Build history of the part. All positions in model axes, mm. A direction names the side the tool comes from. Round coordinates to 2 decimals unless told otherwise and drop trailing zeros. Order: outer loops, then holes, each group sorted by start corner. A loop starts at its lowest first (then second) coordinate and runs counter-clockwise, first axis right, second up. Notation, with made-up numbers: (21.5, -21) -> (48.5, -21) arc R12 ccw to (48.5, -15) -> close; hole circle Ø3 at (-4.5, 11). An arc over 180 degrees is marked (long way). Use a Markdown table: item, result. Add a question column.
Item 1: Probe L1, parallel to X at y = 3.5, z = 5; L2, parallel to Z at x = 21, y = 5.25 (3 decimals); L3, parallel to Y at x = -2.5, z = 3.5. List the from-to ranges inside material, lowest first.
Item 2: 3-axis set-ups, long thin cutter, end or side, ignore diameter. For faces 5 (the face through (2, 7.525, 2)), 6 (the face through (-2, 0, 7.264)), 7 (the face through (-27.43, 2.47, 4.58)): which of +Z, -Z, +X, -X, +Y, -Y reach the whole face in a straight line?
Item 3: Two-plate mould, pull along X, no slides. Class faces 1 (the face through (-36.528, 4, 2)), 2 (the face through (-5.701, 3.284, 5.066)), 3 (the face through (39.672, 1, 2)), 4 (the face through (30, -1, 9.093)): released by +X, released by -X, zero draft, split by the parting line, or undercut.
Item 4: Pin check, flat tips, straight feed: pin 1 (1.7 mm diameter, centred on x = -31.5, y = 2, fed in from +Z); pin 2 (3 mm diameter, centred on x = -22.5, y = 4.5, fed in from +Z) (3 decimals); pin 3 (8 mm diameter, centred on x = -17.5, y = 3, fed in from +Z) (3 decimals); pin 4 (8 mm diameter, centred on x = -8.5, y = 5.5, fed in from -Z). Stop position of each tip, or through.
Item 5: Slice it at C-C, the plane y = -9.25. Give the cut face in (x, z) (3 decimals), plus the area to 3 significant figures.
Item 6: Slice it at A-A, the plane z = 5. Give the cut face in (x, y), plus the area to 3 significant figures.
Item 7: Slice it at B-B, the plane x = 20. Give the cut face in (y, z) (3 decimals), plus the area to 3 significant figures.
from build123d import *

# Parameters (mm, degrees)
F2_R     = 3.1496
F2_R_2   = 4.699
F2_R_3   = 3.8862
F2_R_4   = 5.4864
F2_R_5   = 6.2865
F3_DEPTH = 3.175
F1_R     = 6.2865
F4_DEPTH = 9.0932
F0_R     = 5.4864
F5_DEPTH = 8.6868
F6_DEPTH = 7.2644
F7_DEPTH = 6.985
F8_DEPTH = 6.2738
F9_R     = 5.08
F10_R    = 0.254


with BuildPart() as f3:
    # F2 (on face) → F3 (new body)
    with BuildSketch(Plane.XY):
        Polygon((-36.528022, 7.525173), (-36.528022, -3.904827), (39.671978, -11.524827), (39.671978, 7.525173), align=None)
        with Locations((-30.432022, 1.520613)):
            Circle(F2_R, mode=Mode.SUBTRACT)
        with Locations((-2.238022, 0.108373)):
            Circle(F2_R_2, mode=Mode.SUBTRACT)
        with Locations((-17.224022, 0.921173)):
            Circle(F2_R_3, mode=Mode.SUBTRACT)
        with Locations((13.459178, -0.666327)):
            Circle(F2_R_4, mode=Mode.SUBTRACT)
        with Locations((30.146978, -1.504527)):
            Circle(F2_R_5, mode=Mode.SUBTRACT)
        with Locations((30.146978, -1.504527)):
            Circle(F2_R_5)
        with Locations((13.459178, -0.666327)):
            Circle(F2_R_4)
        with Locations((-2.238022, 0.108373)):
            Circle(F2_R_2)
        with Locations((-17.224022, 0.921173)):
            Circle(F2_R_3)
        with Locations((-30.432022, 1.520613)):
            Circle(F2_R)
    extrude(amount=F3_DEPTH)

    # F1 (on face) → F4 (join)
    with BuildSketch(Plane.XY):
        with Locations((30.146978, -1.504527)):
            Circle(F1_R)
    extrude(amount=F4_DEPTH)

    # F0 (on Top) → F5 (join)
    with BuildSketch(Plane.XY):
        with Locations((13.459178, -0.666327)):
            Circle(F0_R)
    extrude(amount=F5_DEPTH)

    # F2 (on face) → F6 (join)
    with BuildSketch(Plane.XY):
        with Locations((-2.238022, 0.108373)):
            Circle(F2_R_2)
    extrude(amount=F6_DEPTH)

    # F2 (on face) → F7 (join)
    with BuildSketch(Plane.XY):
        with Locations((-17.224022, 0.921173)):
            Circle(F2_R_3)
    extrude(amount=F7_DEPTH)

    # F2 (on face) → F8 (join)
    with BuildSketch(Plane.XY):
        with Locations((-30.432022, 1.520613)):
            Circle(F2_R)
    extrude(amount=F8_DEPTH)

    # F9
    f9_edges = [f3.edges().sort_by_distance(p)[0] for p in [
        (39.671978, -11.524827, 1.5875),
        (-36.528022, -3.904827, 1.5875),
    ]]
    fillet(f9_edges, radius=F9_R)

    # F10
    f10_edges = [f3.edges().sort_by_distance(p)[0] for p in [
        (23.860478, -1.504527, 9.0932),
        (7.972778, -0.666327, 8.6868),
        (-6.937022, 0.108373, 7.2644),
        (-21.110222, 0.921173, 6.985),
        (-33.581622, 1.520613, 6.2738),
    ]]
    fillet(f10_edges, radius=F10_R)


solid = f3.part
Check sheet entries:
| question | item | result |
|---|---|---|
| 1 | L1 | -32.88 to -27.98, -20.13 to -14.32, -5.49 to 1.01, 9.89 to 17.03, 26.34 to 33.95 |
| 1 | L2 | 0 to 3.175 |
| 1 | L3 | -4.58 to 4.8 |
| 2 | face 5 | +Z, -Z, +X, -X, +Y |
| 2 | face 6 | +Z, -X, +Y, -Y |
| 2 | face 7 | +Z |
| 3 | face 1 | released by -X |
| 3 | face 2 | undercut |
| 3 | face 3 | released by +X |
| 3 | face 4 | zero draft |
| 4 | pin 1 | z = 6.27 |
| 4 | pin 2 | z = 3.175 |
| 4 | pin 3 | z = 6.985 |
| 4 | pin 4 | z = 0 |
| 5 | outline | (16.924, 0) -> (38.421, 0) -> (38.421, 3.175) -> (16.924, 3.175) -> close |
| 5 | area | 68.3 mm2 |
| 6 | outline | circle Ø6.3 at (-30.43, 1.52); circle Ø7.77 at (-17.22, 0.92); circle Ø9.4 at (-2.24, 0.11); circle Ø10.97 at (13.46, -0.67); circle Ø12.57 at (30.15, -1.5) |
| 6 | area | 367 mm2 |
| 7 | outline | (-9.558, 0) -> (7.525, 0) -> (7.525, 3.175) -> (-9.558, 3.175) -> close |
| 7 | area | 54.2 mm2 |
